Autodesk Inventor part; units mm, degrees
ref_plane "YZ Plane" through (0, 0, 0) normal (1, 0, 0) x (0, 1, 0)
ref_plane "XZ Plane" through (0, 0, 0) normal (0, 1, 0) x (-1, 0, 0)
ref_plane "XY Plane" through (0, 0, 0) normal (0, 0, 1) x (1, 0, 0)
sketch "Sketch1" plane through (0, 0, 0) normal (0, 0, 1) x (1, 0, 0)
  line L0 (0, 0) -> (2235.2, 0)
  line L1 (0, 0) -> (218.4618, -102.4702)
  line L2 (2235.2, 0) -> (2016.7382, -102.4702)
  line L3 (218.4618, -102.4702) -> (2016.7382, -102.4702)
  line L4 (1016.751, -102.4702) -> (1016.751, -305.6702)
  line L5 (1016.751, -305.6702) -> (1067.551, -305.6702)
  line L6 (1067.551, -305.6702) -> (1067.551, -102.4702)
  dimension "d1" = 2235.2
  dimension "d2" = 241.3
  dimension "d3" = 241.3
  dimension "d7" = 203.2
  dimension "d8" = 50.8
extrude "Extrusion1" add sketch "Sketch1" along normal blind 1219.2 contours L0 L2 L3 L1
properties part number "Bridge"
Model file for the job. Use its own axes, mm. Round coordinates to 2 decimals unless told otherwise and drop trailing zeros. Order: outer loops, then holes, each group sorted by start corner. A loop starts at its lowest first (then second) coordinate and runs counter-clockwise, first axis right, second up. Notation, with made-up numbers: M -18,14.25 L 0,14.25 A17 cw 0,41.25 Z; hole C 19.25,-10.5 d6. An arc over 180 degrees is marked long. Use CSV: the item, a comma, the result in double quotes.
Item 1: Probe probe 1 along X at (y, z) = (-47, 481); probe 2 along X at (y, z) = (-20.5, 430); probe 3 along Y at (x, z) = (2143, 1097.5). List the from-to ranges inside material, lowest first.
Worked answers:
probe 1,"100.2 to 2135"
probe 2,"43.71 to 2191.49"
probe 3,"-43.25 to 0"
Item 2: Saw through at A-A (z = 723.5). List the corners of the cut face in (x, y).
Worked answers:
outline,"M 0,0 L 218.46,-102.47 L 2016.74,-102.47 L 2235.2,0 Z"
Item 3: Pin check, flat tips, straight feed: pin 1 (8 mm diameter, centred on y = -80.5, z = 644, fed in from -X); pin 2 (8 mm diameter, centred on y = -10.5, z = 668, fed in from -X); pin 3 (5 mm diameter, centred on y = -16.5, z = 852.5, fed in from +X). Stop position of each tip, or through.
Worked answers:
pin 1,"x = 163.09"
pin 2,"x = 13.86"
pin 3,"x = 2205.35"
Item 4: Saw through at B-B (y = -42). List the corners of the cut face in (x, z).
Worked answers:
outline,"M 89.54,0 L 2145.66,0 L 2145.66,1219.2 L 89.54,1219.2 Z"
